Verification items for this drawing (mm, ordinates from the low corner). Coordinates: 2 decimals unless noted, no trailing zeros. Order: outer loops, then holes, each group sorted by start corner. A loop starts at its lowest first (then second) coordinate and runs counter-clockwise, first axis right, second up. Notation, with made-up numbers: (73, 41.5) -> (94, 41.5) arc R13 ccw to (94, 53.5) -> close; hole circle Ø5 at (-35.75, 58.5). An arc over 180 degrees is marked (long way). Answer in a Markdown table with one row per item. Add a question column.
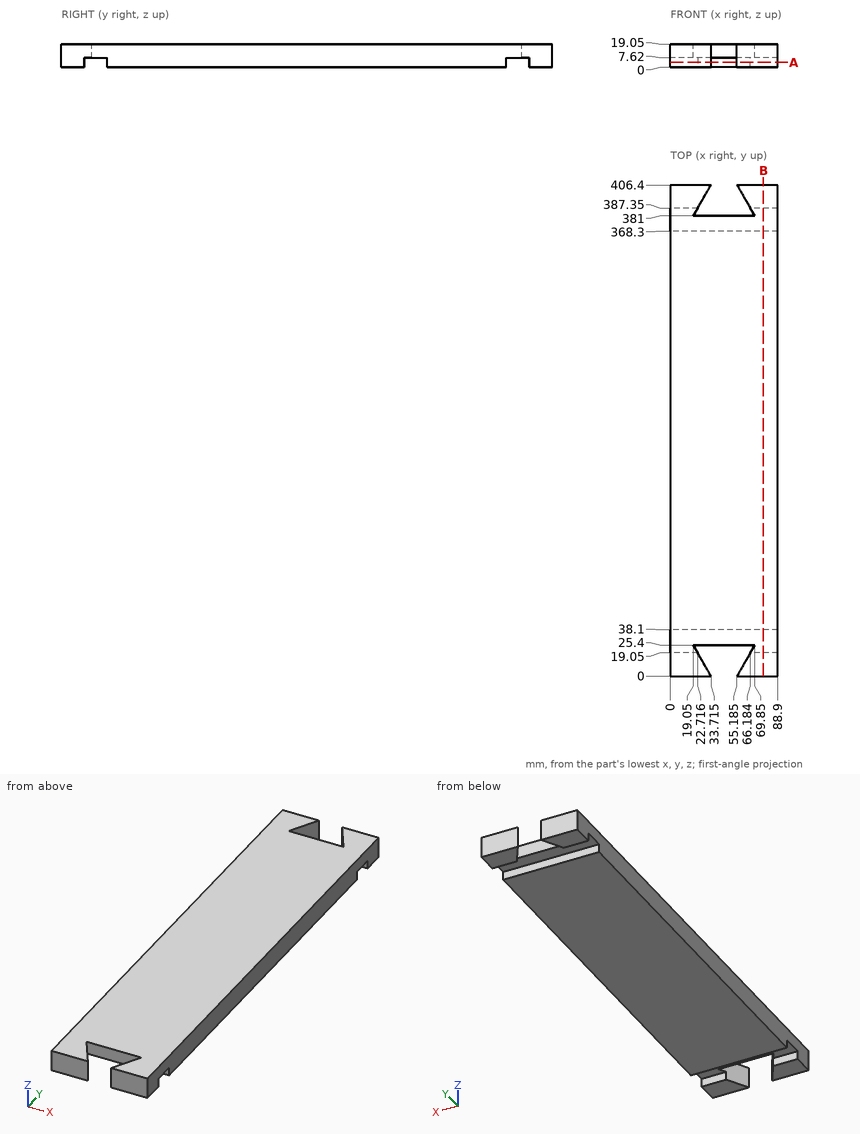
(1) Cross-section at A-A (z = 3.75). Give the number of separate pieces and of enclosed holes in the cut face, plus the area to 3 significant figures.
(2) Scan lines: line 1 along Y through (x, z) = (22, 5.5); line 2 along Y through (x, z) = (22, 8); line 3 along Y through (x, z) = (52, 3.25). Record each from-to range of solid material in increasing order.
(3) Cross-section at B-B (x = 77). Enter the section's corners in (y, z), plus the area to 3 significant figures.
(4) Go/stop test with flat-tipped pins: P1, Ø21, axis at x = 35.5, y = 381, coming from the -Z side; P2, Ø1.5, axis at x = 45.5, z = 14, coming from the -Y side. Record where each tip stops, or that it passes through.
Checks:
| question | item | result |
|---|---|---|
| 1 | separate pieces | 5 |
| 1 | enclosed holes | 0 |
| 1 | area | 31,500 mm² |
| 2 | line 1 | 0 to 19.05, 38.1 to 368.3, 387.35 to 406.4 |
| 2 | line 2 | 0 to 20.29, 25.4 to 381, 386.11 to 406.4 |
| 2 | line 3 | 38.1 to 368.3 |
| 3 | outline | (0, 0) -> (19.05, 0) -> (19.05, 7.62) -> (38.1, 7.62) -> (38.1, 0) -> (368.3, 0) -> (368.3, 7.62) -> (387.35, 7.62) -> (387.35, 0) -> (406.4, 0) -> (406.4, 19.05) -> (0, 19.05) -> close |
| 3 | area | 7,450 mm² |
| 4 | P1 | z = 7.62 |
| 4 | P2 | y = 25.4 |
